Autodesk Fusion 360 part; units mm, degrees
sketch "Sketch1" plane through (0, 0, 0) normal (0, 0, 1) x (1, 0, 0)
  circle A0 centre (0, 0) radius 90
  circle A1 centre (0, 65) radius 10
  circle A2 centre (0, -65) radius 10
  circle A3 centre (0, 0) radius 25
  circle A4 centre (0, 0) radius 35
  circle A5 centre (0, 65) radius 20
  circle A6 centre (0, -65) radius 20
  line L0 (-10, 30) -> (10, 30)
  line L1 (10, 30) -> (10, 50)
  line L2 (10, 50) -> (-10, 50)
  line L3 (-10, 50) -> (-10, 30)
  line L4 (-10, -30) -> (10, -30)
  line L5 (10, -30) -> (10, -50)
  line L6 (10, -50) -> (-10, -50)
  line L7 (-10, -50) -> (-10, -30)
  dimension "d1" = 50
extrude "Extrude1" add sketch "Sketch1" along normal blind 5 contours A4 L0 L1 L3 L4 L5 L7 | A4 L0 L1 L3 | A4 A5 L1 L3 | A4 A6 L5 L7 | A4 L4 L5 L7 | A5 L1 L2 L3 | A5 L1 L2 L3 | A6 L5 L6 L7 | A6 L5 L6 L7 makes body 1
sketch "Sketch2" plane through (0, 0, 0) normal (0, 0, 1) x (1, 0, 0)
sketch "Sketch3" plane through (0, 0, 0) normal (0, 0, 1) x (1, 0, 0)
  circle A0 centre (0, 0) radius 30
extrude "Extrude2" cut sketch "Sketch3" along normal blind 8 bodies 1
sketch "Sketch4" plane through (0, 0, 0) normal (0, 0, 1) x (1, 0, 0)
sketch "Sketch5" plane through (0, 0, 0) normal (0, 1, 0) x (1, 0, 0)
sketch "Sketch6" plane through (0, 0, 0) normal (0, 0, 1) x (1, 0, 0)
  circle A0 centre (0, 65) radius 5.25
  circle A1 centre (0, 65) radius 10
  dimension "d6" = 10.5
extrude "Extrude3" add sketch "Sketch6" along normal blind 5 bodies 1
sketch "Sketch7" plane through (0, 0, 0) normal (0, 0, 1) x (1, 0, 0)
  circle A0 centre (0, -65) radius 5.25
  circle A1 centre (0, -65) radius 10
  dimension "d9" = 10.5
extrude "Extrude4" add sketch "Sketch7" along normal blind 5 bodies 1
sketch "Sketch8" plane through (0, 0, 0) normal (0, 0, 1) x (1, 0, 0)
  circle A0 centre (0, 0) radius 40
  circle A1 centre (0, 0) radius 30
  circle A2 centre (0, 0) radius 30
extrude "Extrude5" add sketch "Sketch8" along normal blind 5 bodies 1
sketch "Sketch9" plane through (0, 0, 0) normal (0, 0, 1) x (1, 0, 0)
sketch "Sketch10" plane through (0, 0, 0) normal (0, 0, 1) x (1, 0, 0)
sketch "Sketch11" plane through (0, 0, 0) normal (0, 0, 1) x (1, 0, 0)
sketch "Sketch12" plane through (0, 0, 0) normal (0, 0, 1) x (1, 0, 0)
  circle A0 centre (0, 65) radius 15
  circle A1 centre (0, 65) radius 20
extrude "Extrude6" cut sketch "Sketch12" along normal blind 30 bodies 1 makes body 2 at (11.6746, 63.994, 0)
sketch "Sketch13" plane through (0, 0, 0) normal (0, 0, 1) x (1, 0, 0)
  circle A0 centre (0, -65) radius 15
  circle A1 centre (0, -65) radius 20
extrude "Extrude7" cut sketch "Sketch13" along normal blind 22 bodies 1 makes body 3 at (3.3287, -53.7649, 0)
sketch "Sketch14" plane through (0, 0, 0) normal (0, 0, 1) x (1, 0, 0)
  line L0 (-10, -35) -> (10, -35)
  line L1 (10, -35) -> (10, -59)
  line L2 (10, -59) -> (-10, -59)
  line L3 (-10, -59) -> (-10, -35)
  line L4 (-10, 35) -> (10, 35)
  line L5 (10, 35) -> (10, 58)
  line L6 (10, 58) -> (-10, 58)
  line L7 (-10, 58) -> (-10, 35)
extrude "Extrude8" add sketch "Sketch14" along normal blind 5 bodies 1 2 3
Could you check a few things on this model? Use its own coordinates, in mm. A direction names the side the tool comes from. Give positions to 0.01 mm unless a question says otherwise; leave off trailing zeros. Order: outer loops, then holes, each group sorted by start corner. A loop starts at its lowest first (then second) coordinate and runs counter-clockwise, first axis right, second up. Notation, with made-up numbers: (-6, 81) - (50, 81) arc R20 ccw to (50, 119) - close; hole circle Ø6 at (-7, -24). An arc over 180 degrees is marked (long way). One line per question, with ' | ' between items. Start each with the question number.
Item 1: I need wall thicknesses on probe 1 along Y at (x, z) = (0.5, 3); probe 2 along Y at (x, z) = (12, 3.5); probe 3 along Y at (x, z) = (23, 1.95). Which ranges of each line are inside material? Lowest first, please. Write a range as [from, to].
Item 2: For faces 1 (the flat face through (10, -46, 2)), 2 (the flat face through (-10, -46, 2)), 3 (the cylindrical face through (2.42, -60.34, 2.46)), which set-ups out of +Z, -Z, +X, -X, +Y, -Y let a thin tool reach every point of the face, with its end or its side?
Item 3: I want a section at B-B on x = 20.5. Write out the boundary of the cut face in (y, z), then the cut area to 3 significant figures.
Item 4: I want a section at C-C on z = 3. Write out the boundary of the cut face in (x, y), then the cut area to 3 significant figures.
Item 5: I want a section at D-D on y = 43.5. Write out the boundary of the cut face in (x, z), then the cut area to 3 significant figures.
Item 6: I want a section at A-A on y = 0. Write out the boundary of the cut face in (x, z).
Item 7: Thinking about a two-plate mould opening in X: for faces 4 (the flat face through (-10, 46, 2)), 5 (the cylindrical face through (39.993, 0.738, 2.465)), 6 (the cylindrical face through (-29.97, -1.32, 2.46)), 7 (the flat face through (-30, 6, 5)), which applies, pulls with the +X half, pulls with the -X half, needs draft (parallel to the pull), parting line crosses it, or undercut?
Item 8: I'm going to push flat-ended pins straight in: pin 1 Ø8.5 at (x, y) = (0, -65) entering from -Z; pin 2 Ø1 at (x, z) = (11, 3.5) entering from -Y; pin 3 Ø2.5 at (y, z) = (-48, 1.5) entering from -X. Where does each tip first touch, or does it pass through?
Verdict:
1) probe 1: [-79.99, -70.23], [-59.77, -30], [30, 59.77], [70.23, 79.99] | probe 2: [-74, -56], [-38.16, -27.5], [27.5, 38.16], [56, 74] | probe 3: [-32.73, -19.26], [19.26, 32.73]
2) face 1: +Z, -Z, +X | face 2: +Z, -Z, -X | face 3: +Z, -Z
3) outline: (-34.35, 0) - (-21.9, 0) - (-21.9, 5) - (-34.35, 5) - close; (21.9, 0) - (34.35, 0) - (34.35, 5) - (21.9, 5) - close | area: 124 mm^2
4) outline: (-10, -53.82) arc R15 ccw (long way) to (10, -53.82) - (10, -38.73) arc R40 ccw to (10, 38.73) - (10, 53.82) arc R15 ccw (long way) to (-10, 53.82) - (-10, 38.73) arc R40 ccw to (-10, -38.73) - close; hole circle Ø60 at (0, 0); hole circle Ø10.5 at (0, -65); hole circle Ø10.5 at (0, 65) | area: 3,900 mm^2
5) outline: (-10, 0) - (10, 0) - (10, 5) - (-10, 5) - close | area: 100 mm^2
6) outline: (-40, 0) - (-30, 0) - (-30, 5) - (-40, 5) - close; (30, 0) - (40, 0) - (40, 5) - (30, 5) - close
7) face 4: pulls with the -X half | face 5: pulls with the +X half | face 6: undercut | face 7: needs draft
8) pin 1: through | pin 2: y = -75.71 | pin 3: x = -10
